from build123d import *

# Parameters (mm, degrees)
F0_W     = 9.398
F0_H     = 9.398
F1_DEPTH = 4.699
F5_R     = 6.4204248834
F6_DEPTH = 1.8481535467


with BuildPart() as f1:
    # F0 (on Top) → F1 (new body, symmetric)
    with BuildSketch(Plane.XY):
        with Locations((4.699, 4.699)):
            Rectangle(F0_W, F0_H)
    extrude(amount=F1_DEPTH, both=True)

    # F2 (on Top) → F3 (revolve)
    with BuildSketch(Plane.XY):
        with BuildLine():
            Line((2.1089997974, 4.1338952074), (-42.9354029785, 16.2035065548))
            Line((-42.9354029785, 16.2035065548), (-43.7571534467, 13.1366920563))
            add(Edge.make_bspline(
                [(-43.7571534467, 13.1366920563), (-31.4497982907, 9.7613016894), (-24.351204811, 4.7111827292), (-17.0302603516, 5.3395174522), (-15.1165829072, 5.2838661547)],
                knots=[0, 0, 0, 0, 0.3695067748, 0.5217943897, 0.5217943897, 0.5217943897, 0.5217943897], degree=3))
            add(Edge.make_bspline(
                [(-15.1165829072, 5.2838661547), (-14.2199308743, 5.2577907838), (-12.4153866633, 5.090572736), (-10.9454237567, 4.3486670485), (-10.2269043728, 3.911686346)],
                knots=[0.5217943897, 0.5217943897, 0.5217943897, 0.5217943897, 0.5931486296, 0.6736895744, 0.6736895744, 0.6736895744, 0.6736895744], degree=3))
            add(Edge.make_bspline(
                [(-10.2269043728, 3.911686346), (-9.3735957348, 3.3927310938), (-6.755614661, 1.4125647276), (-4.4911950827, 1.0167984292), (1.2996370206, 1.1133122025)],
                knots=[0.6736895744, 0.6736895744, 0.6736895744, 0.6736895744, 0.769339442, 1, 1, 1, 1], degree=3))
            Line((1.2996370206, 1.1133122025), (2.1089997974, 4.1338952074))
        make_face()
        with BuildLine():
            add(Edge.make_bspline(
                [(-15.1165829072, 5.2838661547), (-14.2199308743, 5.2577907838), (-12.4153866633, 5.090572736), (-10.9454237567, 4.3486670485), (-10.2269043728, 3.911686346)],
                knots=[0.5217943897, 0.5217943897, 0.5217943897, 0.5217943897, 0.5931486296, 0.6736895744, 0.6736895744, 0.6736895744, 0.6736895744], degree=3))
            ThreePointArc((-15.1165829072, 5.2838661547), (-12.9898277475, 3.4643030547), (-10.2269043728, 3.911686346))
        make_face()
    revolve(axis=Axis((-20.4132015906, 10.1687008811, 0), (0.9659258263, -0.2588190451, 0)))

    # F5 (on offset) → F6 (cut, through all)
    with BuildSketch(Plane.YZ.offset(-41.91)):
        with Locations((16.1998961121, 0)):
            Circle(F5_R)
    extrude(amount=-F6_DEPTH, mode=Mode.SUBTRACT)


solid = f1.part
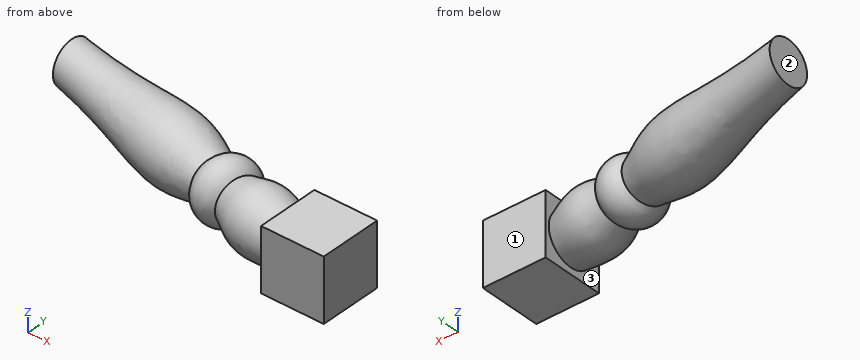
Input: part model. Units: mm. Frame: model coordinates. Face numbers are marked on the shaded views. A direction names the side the tool comes from. Give positions to 0.01 mm unless a question says otherwise; leave off trailing zeros. Write each loop counter-clockwise with the first axis right and the second up, starting at its lowest first coordinate (ties: lowest second). Pieces come first, ordered by that corner, then holes. Notation, with made-up numbers: (60, 77) -> (73, 77) arc R22 cw to (73, 109) -> close; hole circle Ø4 at (-36, 19). An arc over 180 degrees is marked (long way). Use one line per item in the form item = value. Start each with the question number.
1) Pin query (flat end, axial travel): pin 1 (3 mm diameter, centred on x = 3, y = 3, fed in from -Z); pin 2 (7.5 mm diameter, centred on x = 3, y = 3, fed in from +Z); pin 3 (10 mm diameter, centred on x = -11, y = 12, fed in from -Z). Return the tip coordinate at first contact, or that it passes through.
2) Set-up query: the marked faces 1, 2 and 3. Return all of +Z, -Z, +X, -X, +Y, -Y with unobstructed straight access to the full face (end or side cutting, diameter ignored); none if empty.
3) Ray query, probe 1 along X at (y, z) = (9, 1.75); probe 2 along Z at (x, y) = (-20, 8.75); probe 3 along Z at (x, y) = (6, 3.5). Return the intervals inside material, ascending. Write a range as from..to.
4) Section query A-A on x = 5. Return the cut outline in (y, z), then the cut area to 3 significant figures.
Outcome:
q1.pin_1 = -4.7
q1.pin_2 = 4.7
q1.pin_3 = -4.55
q2.face_1 = +Z, -Z, +X, +Y
q2.face_2 = +Z, -Z, -X, +Y, -Y
q2.face_3 = none
q3.probe_1 = -30.52..-1.09, 0..9.4
q3.probe_2 = -4.55..4.55
q3.probe_3 = -4.7..4.7
q4.outline = (0, -4.7) -> (9.4, -4.7) -> (9.4, 4.7) -> (0, 4.7) -> close
q4.area = 88.3 mm^2
